```python
from build123d import *

# Parameters (mm, degrees)
REVOLVE_2_ANGLE = 270
EXTRUDE_1_DEPTH = 120


with BuildPart() as part:
    # 草图2 → 旋转2 (revolve)
    with BuildSketch(Plane(origin=(0, 0, 0), x_dir=(1, 0, 0), z_dir=(0, 1, 0))):
        with BuildLine():
            Line((-34.5, 0), (-34.5, 3))
            Line((-34.5, 3), (-43, 3))
            Line((-43, 3), (-43.995557857, 3))
            ThreePointArc((-43.995557857, 3), (-40.98437005, 16.275457684), (-34.067713618, 28))
            Line((-34.067713618, 28), (-35, 28))
            Line((-35, 28), (-35, 30))
            ThreePointArc((-35, 30), (-42.690748412, 17.392527131), (-46, 3))
            Line((-46, 3), (-46, 0))
            Line((-46, 0), (-34.5, 0))
        make_face()
    revolve(axis=Axis((0, 0, -42), (0, 0, 1)), revolution_arc=REVOLVE_2_ANGLE)

    # 草图2<2> → 凸台-拉伸1 (add)
    with BuildSketch(Plane(origin=(0, 0, 0), x_dir=(1, 0, 0), z_dir=(0, 1, 0))):
        with BuildLine():
            Line((-34.5, 0), (-34.5, 3))
            Line((-34.5, 3), (-43, 3))
            Line((-43, 3), (-43.995557857, 3))
            ThreePointArc((-43.995557857, 3), (-40.98437005, 16.275457684), (-34.067713618, 28))
            Line((-34.067713618, 28), (-35, 28))
            Line((-35, 28), (-35, 30))
            ThreePointArc((-35, 30), (-42.690748412, 17.392527131), (-46, 3))
            Line((-46, 3), (-46, 0))
            Line((-46, 0), (-34.5, 0))
        make_face()
    extrude(amount=EXTRUDE_1_DEPTH)


solid = part.part
```
Geometry check sheet. Reference: the model listing, model coordinates, mm. A direction names the side the tool comes from. Coordinates: 2 decimals unless noted, no trailing zeros. Order: outer loops, then holes, each group sorted by start corner. A loop starts at its lowest first (then second) coordinate and runs counter-clockwise, first axis right, second up. Notation, with made-up numbers: M 25.5,-39.5 L 48.5,-39.5 A21 cw 48.5,-15.5 Z; hole C 4.25,64 d7. An arc over 180 degrees is marked long. One line per question, with ' | ' between items. Start each with the question number.
Item 1: Cross-section at C-C on y = 58. Enter the section's corners in (x, z).
Item 2: Material ranges on L1, parallel to X at y = 0, z = -1.2; L2, parallel to Z at x = 2, y = 37; L3, parallel to Y at x = 15, z = -22, recorded low to high. Write a range as [from, to].
Item 3: Cross-section at B-B on x = 15. Enter the section's corners in (y, z).
Item 4: Cross-section at A-A on y = 26. Enter the section's corners in (x, z).
Item 5: Cross-section at D-D on x = -15. Enter the section's corners in (y, z), then the cut area to 3 significant figures.
Item 6: Draft check along Y on faces 4 (the cylindrical face through (23.577, -25.186, -1.521)), 5 (the flat face through (-46, 59, -2)), 6 (the flat face through (-43, 120, -12)). Enter one of: pulls with the +Y half, pulls with the -Y half, needs draft (parallel to the pull), parting line crosses it, or undercut.
Item 7: Set-up check for faces 1 (the cylindrical face through (-41.055, 59.16, -16.097)), 2 (the cylindrical face through (23.92, -25.55, -29.01)), 3 (the flat face through (3, 38, -3)): record each of +Z, -Z, +X, -X, +Y, -Y from which the full face is reachable in a straight line by a thin tool's end or side.
Item 8: Gauge pin test, flat ends, axial feed: pin 1 (6 mm diameter, centred on x = 8.5, z = -11.5, fed in from +Y); pin 2 (2.5 mm diameter, centred on y = 33.5, z = -1, fed in from +X); pin 3 (10 mm diameter, centred on y = -2, z = -24, fed in from +X). Record the tip position at first contact, or that the pin passes through.
Findings:
1) outline: M -46,-3 A46.1 ccw -35,-30 L -35,-28 L -34.07,-28 A44.1 cw -44,-3 L -34.5,-3 L -34.5,0 L -46,0 Z
2) L1: x = [-46, -34.5], [34.5, 46] | L2: z = [-27.42, -23.91], [-3, 0] | L3: y = [-37.63, -35.15], [35.15, 37.63]
3) outline: M -43.49,-3 A43.59 ccw -31.62,-30 L -31.62,-28 L -30.59,-28 A41.47 cw -41.36,-3 L -31.07,-3 L -31.07,0 L -43.49,0 Z; M 30.59,-28 L 31.62,-28 L 31.62,-30 A43.59 ccw 43.49,-3 L 43.49,0 L 31.07,0 L 31.07,-3 L 41.36,-3 A41.47 cw Z
4) outline: M -46,-3 A46.1 ccw -35,-30 L -35,-28 L -34.07,-28 A44.1 cw -44,-3 L -34.5,-3 L -34.5,0 L -46,0 Z; M 22.01,-28 L 23.43,-28 L 23.43,-30 A38.07 ccw 37.95,-3 L 37.95,0 L 22.68,0 L 22.68,-3 L 35.49,-3 A35.62 cw Z
5) outline: M -43.49,-3 A43.59 ccw -31.62,-30 L -31.62,-28 L -30.59,-28 A41.47 cw -41.36,-3 L -31.07,-3 L -31.07,0 L -43.49,0 Z | area: 97.5 mm²
6) face 4: undercut | face 5: needs draft | face 6: pulls with the +Y half
7) face 1: +Y | face 2: -Z | face 3: none
8) pin 1: stops at y = 44.69 | pin 2: stops at x = 32.8 | pin 3: stops at x = 41.96
